The model under review builds one solid part; all positions refer to its coordinate system, in mm. Face numbers are marked on the shaded views. A direction names the side the tool comes from. Coordinates: 2 decimals unless noted, no trailing zeros. Order: outer loops, then holes, each group sorted by start corner. A loop starts at its lowest first (then second) coordinate and runs counter-clockwise, first axis right, second up. Notation, with made-up numbers: M -28.5,41.25 L 9.5,41.25 A19 ccw 9.5,67.25 Z; hole C -28,8.5 d1. An arc over 180 degrees is marked long. Answer in a Markdown table with one row per item.
Autodesk Inventor part; units mm, degrees
ref_plane "YZ Plane" through (0, 0, 0) normal (1, 0, 0) x (0, 1, 0)
ref_plane "XZ Plane" through (0, 0, 0) normal (0, 1, 0) x (-1, 0, 0)
ref_plane "XY Plane" through (0, 0, 0) normal (0, 0, 1) x (1, 0, 0)
sketch "Skizze1" plane through (0, 0, 0) normal (0, 0, 1) x (1, 0, 0)
  circle A0 centre (0, 0) radius 3.25
  line L0 (-10, -10) -> (10, -10)
  line L1 (10, -10) -> (10, 10)
  line L2 (10, 10) -> (-10, 10)
  line L3 (-10, 10) -> (-10, -10)
  line L4 (-10, -10) -> (10, 10) construction
  line L5 (10, -10) -> (-10, 10) construction
  dimension "d0" = 6.5
  dimension "d1" = 20
extrude "Extrusion1" add sketch "Skizze1" along normal blind 2
sketch "Skizze2" plane through (0, 0, 2) normal (0, 0, 1) x (1, 0, 0)
  line L0 (-8.5, -8.5) -> (8.5, -8.5)
  line L1 (8.5, -8.5) -> (8.5, 8.5)
  line L2 (8.5, 8.5) -> (-8.5, 8.5)
  line L3 (-8.5, 8.5) -> (-8.5, -8.5)
  line L4 (-8.5, -8.5) -> (8.5, 8.5) construction
  line L5 (8.5, -8.5) -> (-8.5, 8.5) construction
  circle A0 centre (0, 0) radius 3.25
  dimension "d4" = 17
extrude "Extrusion2" add sketch "Skizze2" along normal blind 15
sketch "Skizze3" plane through (0, 0, 17) normal (0, 0, 1) x (1, 0, 0)
  line L0 (0, 4.6188) -> (4, 2.3094)
  line L1 (4, 2.3094) -> (4, -2.3094)
  line L2 (4, -2.3094) -> (0, -4.6188)
  line L3 (0, -4.6188) -> (-4, -2.3094)
  line L4 (-4, -2.3094) -> (-4, 2.3094)
  line L5 (-4, 2.3094) -> (0, 4.6188)
  point P0 (0, 0)
  point P1 (0, 0)
  dimension "d7" = 8
extrude "Extrusion3" cut sketch "Skizze3" against normal blind 5
properties part number "AlutubeMount"
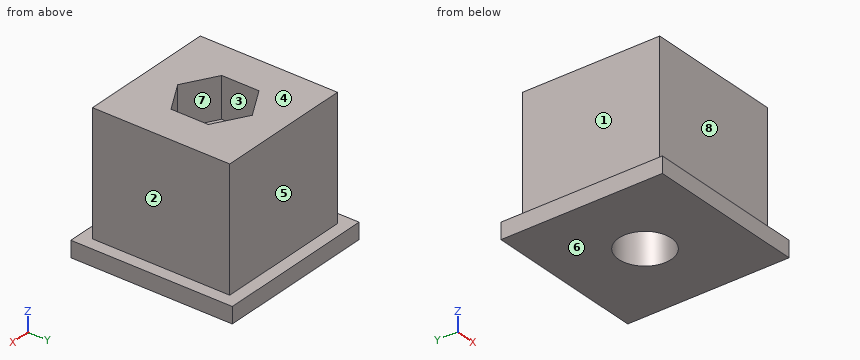
(1) Machinability: for the marked faces 5, 6, 7 and 8, which of the approach directions +Z, -Z, +X, -X, +Y, -Y give a long, thin tool a straight path to every point of the face, cutting with its end or side? Answer none if there is none.
Report:
| item | result |
|---|---|
| face 5 | +Z, +X, -X, +Y |
| face 6 | -Z, +X, -X, +Y, -Y |
| face 7 | +Z |
| face 8 | +Z, +X, -X, -Y |
(2) Take a section at C-C (x = -1.75). Write out the cut boundary in (y, z), then the cut area to 3 significant figures.
Report:
| item | result |
|---|---|
| outline | M -10,0 L -2.74,0 L -2.74,12 L -3.61,12 L -3.61,17 L -8.5,17 L -8.5,2 L -10,2 Z; M 2.74,0 L 10,0 L 10,2 L 8.5,2 L 8.5,17 L 3.61,17 L 3.61,12 L 2.74,12 Z |
| area | 193 mm^2 |
(3) To check wall thickness, follow line 1 (Y direction, x = 0, z = 6.5); line 2 (X direction, y = 0, z = 13). State the ranges of each line that lie inside material, in increasing order. Write a range as [from, to].
Report:
| item | result |
|---|---|
| line 1 | [-8.5, -3.25], [3.25, 8.5] |
| line 2 | [-8.5, -4], [4, 8.5] |
(4) Take a section at D-D (x = -7.75). Write out the cut boundary in (y, z).
Report:
| item | result |
|---|---|
| outline | M -10,0 L 10,0 L 10,2 L 8.5,2 L 8.5,17 L -8.5,17 L -8.5,2 L -10,2 Z |
(5) Take a section at B-B (z = 10.5). Write out the cut boundary in (x, y), then the cut area to 3 significant figures.
Report:
| item | result |
|---|---|
| outline | M -8.5,-8.5 L 8.5,-8.5 L 8.5,8.5 L -8.5,8.5 Z; hole C 0,0 d6.5 |
| area | 256 mm^2 |
(6) Take a section at A-A (y = 0). Write out the cut boundary in (x, z), then the cut area to 3 significant figures.
Report:
| item | result |
|---|---|
| outline | M -10,0 L -3.25,0 L -3.25,12 L -4,12 L -4,17 L -8.5,17 L -8.5,2 L -10,2 Z; M 3.25,0 L 10,0 L 10,2 L 8.5,2 L 8.5,17 L 4,17 L 4,12 L 3.25,12 Z |
| area | 177 mm^2 |
(7) The part is to be moulded in two halves that separate along X. For the marked faces 1, 2, 3 and 4, say which applies: +X half, -X half, draft (parallel to the pull), parting line (faces both ways), or undercut.
Report:
| item | result |
|---|---|
| face 1 | -X half |
| face 2 | +X half |
| face 3 | undercut |
| face 4 | draft |
(8) Insertion check: P1, Ø1.4, axis at y = 1, z = 13.5, coming from the -X side; P2, Ø4.5, axis at x = -2, z = 10, coming from the -Y side; P3, Ø5, axis at y = -0.5, z = 15.5, coming from the +X side; P4, Ø4, axis at x = 0, y = 0, coming from the +Z side. Each pin has a flat end and moves straight along its axis. Give the tip position at first contact, or say it passes through.
Report:
| item | result |
|---|---|
| P1 | x = -8.5 |
| P2 | y = -8.5 |
| P3 | x = 8.5 |
| P4 | through |
